Model file for the job. Use its own axes, mm. A direction names the side the tool comes from. Round coordinates to 2 decimals unless told otherwise and drop trailing zeros. Write each loop counter-clockwise with the first axis right and the second up, starting at its lowest first coordinate (ties: lowest second). Pieces come first, ordered by that corner, then holes. Notation, with made-up numbers: (75, 78) - (133, 78) arc R29 ccw to (133, 100) - close; hole circle Ø10 at (-24, 56.5). An arc over 180 degrees is marked (long way). Answer as a JSON object with one key per item and string values. Group by question number.
from build123d import *

# Parameters (mm, degrees)
SKETCH1_R             = 52.5
SKETCH1_R_2           = 40.5
BOSS_EXTRUDE1_DEPTH   = 63
SKETCH2_R             = 17.665
SKETCH2_R_2           = 11.665
BOSS_EXTRUDE2_DEPTH   = 25
BOSS_EXTRUDE2_2_DEPTH = 25
BOSS_EXTRUDE3_DEPTH   = 9
CUT_EXTRUDE1_DEPTH    = 57


with BuildPart() as part:
    # Sketch1 → Boss-Extrude1 (new body)
    with BuildSketch(Plane(origin=(0, 0, 0), x_dir=(1, 0, 0), z_dir=(0, 1, 0))):
        with Locations(Location((0, 0, 0), (0, 0, 270))):
            Circle(SKETCH1_R)
        with Locations(Location((0, 0, 0), (0, 0, 270))):
            Circle(SKETCH1_R_2, mode=Mode.SUBTRACT)
    extrude(amount=BOSS_EXTRUDE1_DEPTH)



with BuildPart() as body_2:
    # Sketch2 → Boss-Extrude2 (new body)
    with BuildSketch(Plane(origin=(0, 25, 0), x_dir=(1, 0, 0), z_dir=(0, 1, 0))):
        with Locations(Location((87.5, 0, 0), (0, 0, 270))):
            Circle(SKETCH2_R)
        with Locations(Location((87.5, 0, 0), (0, 0, 270))):
            Circle(SKETCH2_R_2, mode=Mode.SUBTRACT)
    extrude(amount=-BOSS_EXTRUDE2_DEPTH)


with BuildPart() as body_3:
    # Sketch2 → Boss-Extrude2 2 (new body)
    with BuildSketch(Plane(origin=(0, 25, 0), x_dir=(1, 0, 0), z_dir=(0, 1, 0))):
        with Locations(Location((-87.5, 0, 0), (0, 0, 270))):
            Circle(SKETCH2_R)
        with Locations(Location((-87.5, 0, 0), (0, 0, 270))):
            Circle(SKETCH2_R_2, mode=Mode.SUBTRACT)
    extrude(amount=-BOSS_EXTRUDE2_2_DEPTH)


with BuildPart() as part_1:
    add(part.part)

    add(body_2.part)  # Boss-Extrude3 merges body 2

    add(body_3.part)  # Boss-Extrude3 merges body 3
    # Sketch3 → Boss-Extrude3 (add)
    with BuildSketch(Plane(origin=(0, 0, 0), x_dir=(-1, 0, 0), z_dir=(0, -1, 0))):
        with BuildLine():
            Line((-94.532688857, 16.204737346), (-20.901, 48.160130803))
            ThreePointArc((-20.901, 48.160130803), (-52.5, 0), (-20.901, -48.160130803))
            Line((-20.901, -48.160130803), (-94.532688857, -16.204737346))
            ThreePointArc((-94.532688857, -16.204737346), (-69.835, 0), (-94.532688857, 16.204737346))
        make_face()
        with BuildLine():
            Line((20.901, 48.160130803), (94.532688857, 16.204737346))
            ThreePointArc((94.532688857, 16.204737346), (69.835, 0), (94.532688857, -16.204737346))
            Line((94.532688857, -16.204737346), (20.901, -48.160130803))
            ThreePointArc((20.901, -48.160130803), (52.5, 0), (20.901, 48.160130803))
        make_face()
    extrude(amount=-BOSS_EXTRUDE3_DEPTH)

    # Sketch4 → Cut-Extrude1 (cut)
    with BuildSketch(Plane(origin=(0, 63, 0), x_dir=(1, 0, 0), z_dir=(0, 1, 0))):
        with BuildLine():
            Line((-78.726335185, 19.794191843), (-45.264792214, 34.316156339))
            ThreePointArc((-45.264792214, 34.316156339), (-43.494143933, 33.874471647), (-43.460387791, 32.049878207))
            ThreePointArc((-43.460387791, 32.049878207), (-54, 0), (-43.460387791, -32.049878207))
            ThreePointArc((-43.460387791, -32.049878207), (-43.494143933, -33.874471647), (-45.264792214, -34.316156339))
            Line((-45.264792214, -34.316156339), (-78.726335185, -19.794191843))
            ThreePointArc((-78.726335185, -19.794191843), (-79.628461818, -18.464071905), (-78.809359951, -17.081276315))
            ThreePointArc((-78.809359951, -17.081276315), (-68.335, 0), (-78.809359951, 17.081276315))
            ThreePointArc((-78.809359951, 17.081276315), (-79.628461818, 18.464071905), (-78.726335185, 19.794191843))
        make_face()
        with BuildLine():
            Line((78.726335185, -19.794191843), (45.264792214, -34.316156339))
            ThreePointArc((45.264792214, -34.316156339), (43.494143933, -33.874471647), (43.460387791, -32.049878207))
            ThreePointArc((43.460387791, -32.049878207), (54, 0), (43.460387791, 32.049878207))
            ThreePointArc((43.460387791, 32.049878207), (43.494143933, 33.874471647), (45.264792214, 34.316156339))
            Line((45.264792214, 34.316156339), (78.726335185, 19.794191843))
            ThreePointArc((78.726335185, 19.794191843), (79.628461818, 18.464071905), (78.809359951, 17.081276315))
            ThreePointArc((78.809359951, 17.081276315), (68.335, 0), (78.809359951, -17.081276315))
            ThreePointArc((78.809359951, -17.081276315), (79.628461818, -18.464071905), (78.726335185, -19.794191843))
        make_face()
    extrude(amount=-CUT_EXTRUDE1_DEPTH, mode=Mode.SUBTRACT)


solid = part_1.part
(1) Flat gauge pins, fed straight in: pin 1 (4 mm diameter, centred on x = -76.5, y = 9.5, fed in from -Z); pin 2 (1.5 mm diameter, centred on x = 2.5, y = 55, fed in from +Z); pin 3 (6 mm diameter, centred on x = -55, y = 11, fed in from +Z). Where does each tip first touch, or does it go through?
(2) Slice it at B-B (z = 0). Count the separate pieces of the cut face and the enclosed holes in it, then the cut area to 3 significant figures.
(3) Slice it at A-A (x = 0). Write the cut outline in (y, z).
(4) Slice it at C-C (y = 11). Write the cut outline in (x, z) (3 decimals).
(5) Drill centre lines: line 1 (X direction, y = 16, z = 0) (3 decimals); line 2 (Z direction, x = 87, y = 17); line 3 (X direction, y = 16, z = -8). Where is each one in solid material? Low to high. Write a range as from..to.
(6) Pull direction Z, two halves, no side cores. Call faces 4 (the cylindrical face through (105.015, 15.453, -2.3)), 5 (the flat face through (62, 6, 0)), 6 (the flat face through (57.201, 4.437, 32.406)), 7 (the cylindrical face through (-68.337, 7.521, 0.295)): pulls with the +Z half, pulls with the -Z half, needs draft (parallel to the pull), parting line crosses it, or undercut.
(7) 3-axis set-ups, long thin cutter, end or side, ignore diameter. For faces 1 (the flat face through (-31, 63, 27)), 2 (the cylindrical face through (-104.745, 15.453, -3.829)), 3 (the flat face through (-91, 25, 12)): which of +Z, -Z, +X, -X, +Y, -Y reach the whole face in a straight line?
(8) Slice it at D-D (y = 54.5). Write the cut outline in (x, z).
Answer:
{
 "1": {"pin 1": "z = -24.87", "pin 2": "z = 52.47", "pin 3": "z = 34.33"},
 "2": {"separate pieces": "4", "enclosed holes": "0", "area": "2,340 mm²"},
 "3": {"outline": "(0, -52.5) - (63, -52.5) - (63, -40.5) - (0, -40.5) - close; (0, 40.5) - (63, 40.5) - (63, 52.5) - (0, 52.5) - close"},
 "4": {"outline": "circle Ø35.33 at (-87.5, 0); circle Ø105 at (0, 0); circle Ø35.33 at (87.5, 0); hole circle Ø23.33 at (-87.5, 0); hole circle Ø81 at (0, 0); hole circle Ø23.33 at (87.5, 0)"},
 "5": {"line 1": "-105.165..-99.165, -75.835..-69.835, -52.5..-40.5, 40.5..52.5, 69.835..75.835, 99.165..105.165", "line 2": "-17.66..-11.65, 11.65..17.66", "line 3": "-103.25..-95.99, -79.01..-71.75, -51.89..-39.7, 39.7..51.89, 71.75..79.01, 95.99..103.25"},
 "6": {"face 4": "parting line crosses it", "face 5": "undercut", "face 6": "pulls with the +Z half", "face 7": "undercut"},
 "7": {"face 1": "+Z, -Z, +X, -X, +Y", "face 2": "+Y", "face 3": "+Z, -Z, -X, +Y"},
 "8": {"outline": "circle Ø105 at (0, 0); hole circle Ø81 at (0, 0)"}
}
